Geometry: final body of the model. Coordinates: model frame, mm. Face numbers are marked on the shaded views. A direction names the side the tool comes from. Give positions to 0.01 mm unless a question says otherwise; leave off trailing zeros. Write each loop counter-clockwise with the first axis right and the second up, starting at its lowest first coordinate (ties: lowest second). Pieces come first, ordered by that corner, then holes.
Q1. Draft query along X for the marked faces 1, 2 and 3. Return one class per face: pulls with the +X half, pulls with the -X half, needs draft (parallel to the pull), parting line crosses it, or undercut.
Q2. Cut plane A-A on x = 0. Return the cut outline in (y, z) (3 decimals), plus the area to 3 significant figures.
Q3. Line query: L1, parallel to X at y = 2.9, z = 2.5; L2, parallel to X at y = 0.3, z = 2.5; L3, parallel to Y at x = 1.5, z = 8. Output: solid intervals per line, ascending.
Q4. Cut plane B-B on y = -1.25. Return the cut outline in (x, z), plus the area to 3 significant figures.
Q5. Cut plane C-C on z = 2.25. Count the separate pieces of the cut face and the enclosed holes in it, plus the area to 3 significant figures.
Q6. Cut plane D-D on y = 0.75. Return the cut outline in (x, z), plus the area to 3 significant figures.
Q7. Pin query (flat end, axial travel): pin 1 (1 mm diameter, centred on x = 2, z = 1.5, fed in from +Y); pin 2 (3 mm diameter, centred on x = 1, y = -2, fed in from +Z); pin 3 (1 mm diameter, centred on x = 3, z = -6.5, fed in from -Y). Return the tip coordinate at first contact, or that it passes through.
Q8. Reachability of the marked faces 4, 5, 6, 7 and 8 from +Z, -Z, +X, -X, +Y, -Y: full face, straight path, thin tool, end or side. Return the list, or none.
```python
from build123d import *

# Parameters (mm, degrees)
SKETCH1_R                                      = 9
BOSS_EXTRUDE1_DEPTH                            = 3.5
CSK_FOR_M3_FLAT_HEAD_MACHINE_SCREW1_AT_2_COUNT = 2
CSK_FOR_M3_FLAT_HEAD_MACHINE_SCREW1_AT_2_PITCH = 8.660254038
CSK_FOR_M3_FLAT_HEAD_MACHINE_SCREW1_AT_3_COUNT = 2
CSK_FOR_M3_FLAT_HEAD_MACHINE_SCREW1_AT_3_PITCH = 8.660254038
BOSS_EXTRUDE2_START                            = 3.175
BOSS_EXTRUDE2_DEPTH                            = 3.175
FILLET1_R                                      = 3
SKETCH6_R                                      = 2.5
BOSS_EXTRUDE3_DEPTH                            = 3


with BuildPart() as part:
    # Sketch1 → Boss-Extrude1 (new body)
    with BuildSketch(Plane(origin=(0, 0, 0), x_dir=(1, 0, 0), z_dir=(0, 1, 0))):
        with Locations(Location((0, 0, 0), (0, 0, 270))):
            Circle(SKETCH1_R)
    extrude(amount=BOSS_EXTRUDE1_DEPTH)

    # Sketch3 → CSK for M3 Flat Head Machine Screw1 (revolve, cut)
    with BuildSketch(Plane(origin=(0, 3.5, -5), x_dir=(0, 0, 1), z_dir=(1, 0, 0))):
        Polygon((0, 0), (0, 11.021463052), (1.7, 10), (1.7, 2.45), (3.15, 1), (3.15, 0), align=None)
    csk_for_m3_flat_head_machine_screw1 = revolve(axis=Axis((0, 9.85, -5), (0, -1, 0)), mode=Mode.SUBTRACT)

    # CSK for M3 Flat Head Machine Screw1 at 2: CSK for M3 Flat Head Machine Screw1 ×2
    with Locations(*[Vector(0.5000000000000012, 0, 0.866025403784438) * (i * CSK_FOR_M3_FLAT_HEAD_MACHINE_SCREW1_AT_2_PITCH) for i in range(1, CSK_FOR_M3_FLAT_HEAD_MACHINE_SCREW1_AT_2_COUNT)]):
        add(csk_for_m3_flat_head_machine_screw1, mode=Mode.SUBTRACT)

    # CSK for M3 Flat Head Machine Screw1 at 3: CSK for M3 Flat Head Machine Screw1 ×2
    with Locations(*[Vector(-0.500000000000001, 0, 0.8660254037844382) * (i * CSK_FOR_M3_FLAT_HEAD_MACHINE_SCREW1_AT_3_PITCH) for i in range(1, CSK_FOR_M3_FLAT_HEAD_MACHINE_SCREW1_AT_3_COUNT)]):
        add(csk_for_m3_flat_head_machine_screw1, mode=Mode.SUBTRACT)

    # Sketch5 → Boss-Extrude2 (add)
    with BuildSketch(Plane(origin=(0, 3.5, 0), x_dir=(1, 0, 0), z_dir=(0, 1, 0)).offset(BOSS_EXTRUDE2_START)):
        with BuildLine():
            ThreePointArc((-1.93683052, 2.5158125), (-2.749630657, 1.5875), (-3.147172796, 0.419438184))
            ThreePointArc((-3.147172796, 0.419438184), (-4.044126051, 0.636989552), (-4.965632694, 0.585228118))
            ThreePointArc((-4.965632694, 0.585228118), (-4.330127019, 2.5), (-2.989638764, 4.00775))
            ThreePointArc((-2.989638764, 4.00775), (-2.573712159, 3.183821121), (-1.93683052, 2.5158125))
        make_face()
        with BuildLine():
            ThreePointArc((4.965632694, 0.585228118), (4.044126051, 0.636989552), (3.147172796, 0.419438184))
            ThreePointArc((3.147172796, 0.419438184), (2.749630657, 1.5875), (1.93683052, 2.5158125))
            ThreePointArc((1.93683052, 2.5158125), (2.573712159, 3.183821121), (2.989638764, 4.00775))
            ThreePointArc((2.989638764, 4.00775), (4.330127019, 2.5), (4.965632694, 0.585228118))
        make_face()
        with BuildLine():
            ThreePointArc((-1.97599393, -4.592978118), (-1.470413892, -3.820810672), (-1.210342276, -2.935250684))
            ThreePointArc((-1.210342276, -2.935250684), (0, -3.175), (1.210342276, -2.935250684))
            ThreePointArc((1.210342276, -2.935250684), (1.470413892, -3.820810672), (1.97599393, -4.592978118))
            ThreePointArc((1.97599393, -4.592978118), (0, -5), (-1.97599393, -4.592978118))
        make_face()
    extrude(amount=-BOSS_EXTRUDE2_DEPTH)

    # Fillet1
    # the kernel refuses this fillet: 3 mm, written as the material it adds along each edge
    with BuildSketch(Plane(origin=(0, 3.5, 0), x_dir=(-0.1868450460832527, 0, 0.9823893977207547), z_dir=(0.9823893977207547, 0, 0.1868450460832527))) as fillet1_piece_1_section:
        with BuildLine():
            CenterArc((5 + FILLET1_R, -FILLET1_R), FILLET1_R, 90, 90)
            Line((5, -FILLET1_R), (5, 0))
            Line((5, 0), (5 + FILLET1_R, 0))
        make_face()
    fillet1_piece_1 = revolve(axis=Axis((0, 3.5, 0), (0, -1, 0)), revolution_arc=218.462556698, mode=Mode.PRIVATE)
    fillet1_piece_1 = fillet1_piece_1 - Plane(origin=(-4.330127019, 4.03591181, 2.5), x_dir=(0, 0, 1), z_dir=(0, 1, 0)) * Cylinder(3.15, 33, mode=Mode.PRIVATE)
    fillet1_piece_1 = fillet1_piece_1 - Plane(origin=(0, 4.03591181, -5), x_dir=(0, 0, 1), z_dir=(0, 1, 0)) * Cylinder(3.15, 33, mode=Mode.PRIVATE)
    add(fillet1_piece_1)
    with BuildSketch(Plane(origin=(0, 3.5, 0), x_dir=(0.9441966978762919, 0, -0.3293821423810138), z_dir=(-0.3293821423810138, 0, -0.9441966978762919))) as fillet1_piece_2_section:
        with BuildLine():
            CenterArc((5 + FILLET1_R, -FILLET1_R), FILLET1_R, 90, 90)
            Line((5, -FILLET1_R), (5, 0))
            Line((5, 0), (5 + FILLET1_R, 0))
        make_face()
    fillet1_piece_2 = revolve(axis=Axis((0, 3.5, 0), (0, -1, 0)), revolution_arc=218.462556698, mode=Mode.PRIVATE)
    fillet1_piece_2 = fillet1_piece_2 - Plane(origin=(-4.330127019, 4.035911774, 2.5), x_dir=(0, 0, 1), z_dir=(0, 1, 0)) * Cylinder(3.15, 33, mode=Mode.PRIVATE)
    fillet1_piece_2 = fillet1_piece_2 - Plane(origin=(4.330127019, 4.035911774, 2.5), x_dir=(0, 0, 1), z_dir=(0, 1, 0)) * Cylinder(3.15, 33, mode=Mode.PRIVATE)
    add(fillet1_piece_2)
    with BuildSketch(Plane(origin=(0, 3.5, 0), x_dir=(-0.7573516517930461, 0, -0.6530072553397431), z_dir=(-0.6530072553397431, 0, 0.7573516517930461))) as fillet1_piece_3_section:
        with BuildLine():
            CenterArc((5 + FILLET1_R, -FILLET1_R), FILLET1_R, 90, 90)
            Line((5, -FILLET1_R), (5, 0))
            Line((5, 0), (5 + FILLET1_R, 0))
        make_face()
    fillet1_piece_3 = revolve(axis=Axis((0, 3.5, 0), (0, -1, 0)), revolution_arc=218.462556698, mode=Mode.PRIVATE)
    fillet1_piece_3 = fillet1_piece_3 - Plane(origin=(4.330127019, 4.035911774, 2.5), x_dir=(0, 0, 1), z_dir=(0, 1, 0)) * Cylinder(3.15, 32, mode=Mode.PRIVATE)
    fillet1_piece_3 = fillet1_piece_3 - Plane(origin=(0, 4.035911774, -5), x_dir=(0, 0, 1), z_dir=(0, 1, 0)) * Cylinder(3.15, 32, mode=Mode.PRIVATE)
    add(fillet1_piece_3)

    # Sketch6 → Boss-Extrude3 (add)
    with BuildSketch(Plane.XZ):
        with Locations(Location((0, 0, 0), (0, 0, 90))):
            Circle(SKETCH6_R)
    extrude(amount=BOSS_EXTRUDE3_DEPTH)


solid = part.part
```
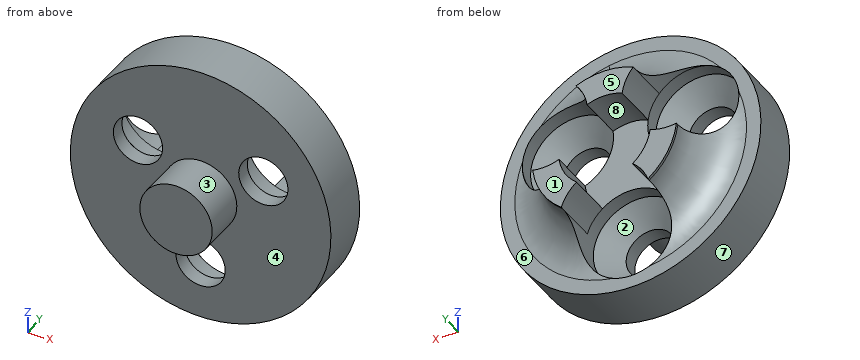
Data:
1. face 1: needs draft
1. face 2: undercut
1. face 3: parting line crosses it
2. outline: (-3, -2.5) - (0, -2.5) - (0, -3.3) - (1.05, -3.3) - (2.5, -1.85) - (3.5, -1.85) - (3.5, 3.175) - (6.675, 3.175) - (6.675, 5) - (6.5, 5) arc R3 cw to (3.5, 8) - (3.5, 9) - (0, 9) - (0, 2.5) - (-3, 2.5) - close; (0, -9) - (3.5, -9) - (3.5, -8.15) - (2.5, -8.15) - (1.05, -6.7) - (0, -6.7) - close
2. area: 68.8 mm2
3. L1: x = -8.65 to -7.48, -1.18 to 1.18, 7.48 to 8.65
3. L2: x = -8.65 to -6.03, -2.63 to 2.63, 6.03 to 8.65
3. L3: y = 0 to 3.5
4. outline: circle Ø5 at (0, 0)
4. area: 19.6 mm2
5. separate pieces: 3
5. enclosed holes: 0
5. area: 33.9 mm2
6. outline: circle Ø18 at (0, 0); hole circle Ø3.4 at (-4.33, 2.5); hole circle Ø3.4 at (0, -5); hole circle Ø3.4 at (4.33, 2.5)
6. area: 227 mm2
7. pin 1: stops at y = 2.39
7. pin 2: stops at z = 2.5
7. pin 3: stops at y = 0
8. face 4: -Y
8. face 5: +Z, -Z, +X, -X, +Y
8. face 6: +Y
8. face 7: +Y, -Y
8. face 8: -Z, +Y
